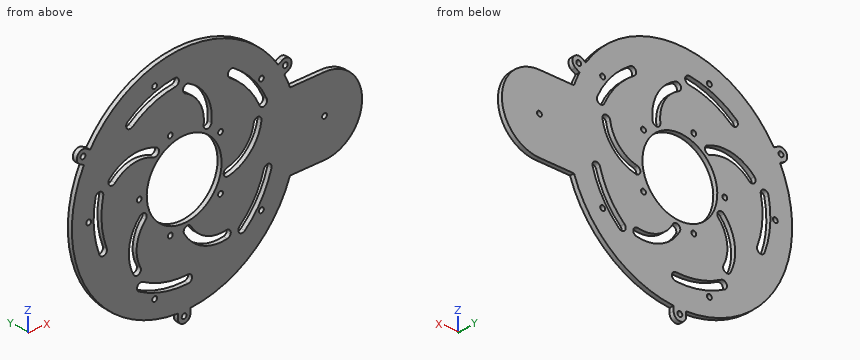
from build123d import *

# Parameters (mm, degrees)
SKETCH1_R           = 50.8
SKETCH1_R_2         = 3.3
BOSS_EXTRUDE1_DEPTH = 6


with BuildPart() as part:
    # Sketch1 → Boss-Extrude1 (new body)
    with BuildSketch(Plane(origin=(0, 0, 0), x_dir=(1, 0, 0), z_dir=(0, 1, 0))):
        with BuildLine():
            Line((190.5, 50.961251532), (143.626985077, 50.961251532))
            ThreePointArc((143.626985077, 50.961251532), (91.342451877, 121.993100154), (8.463835644, 152.16479056))
            Line((8.463835644, 152.16479056), (8.463835644, 158.450241569))
            ThreePointArc((8.463835644, 158.450241569), (0, 166.914077214), (-8.463835644, 158.450241569))
            Line((-8.463835644, 158.450241569), (-8.463835644, 152.16479056))
            ThreePointArc((-8.463835644, 152.16479056), (-131.982271537, 76.2), (-136.010492009, -68.752498599))
            Line((-136.010492009, -68.752498599), (-141.453852257, -71.895224103))
            ThreePointArc((-141.453852257, -71.895224103), (-144.551831116, -83.457038607), (-132.990016613, -86.555017466))
            Line((-132.990016613, -86.555017466), (-127.546656365, -83.412291961))
            ThreePointArc((-127.546656365, -83.412291961), (0, -152.4), (127.546656365, -83.412291961))
            Line((127.546656365, -83.412291961), (132.990016613, -86.555017466))
            ThreePointArc((132.990016613, -86.555017466), (144.551831116, -83.457038607), (141.453852257, -71.895224103))
            Line((141.453852257, -71.895224103), (136.010492009, -68.752498599))
            ThreePointArc((136.010492009, -68.752498599), (140.101433846, -59.977897881), (143.626985077, -50.961251532))
            Line((143.626985077, -50.961251532), (190.5, -50.961251532))
            ThreePointArc((190.5, -50.961251532), (241.461251532, 0), (190.5, 50.961251532))
        make_face()
        with Locations(Location((0, 0, 0), (0, 0, 270))):
            Circle(SKETCH1_R, mode=Mode.SUBTRACT)
        with Locations(Location((-60.96, 0, 0), (0, 0, 270))):
            Circle(SKETCH1_R_2, mode=Mode.SUBTRACT)
        with Locations(Location((-129.54, 0, 0), (0, 0, 270))):
            Circle(SKETCH1_R_2, mode=Mode.SUBTRACT)
        with Locations(Location((-40.030061451, 123.199861121, 0), (0, 0, 270))):
            Circle(SKETCH1_R_2, mode=Mode.SUBTRACT)
        with Locations(Location((-18.837675977, 57.976405233, 0), (0, 0, 270))):
            Circle(SKETCH1_R_2, mode=Mode.SUBTRACT)
        with Locations(Location((104.800061451, 76.141701582, 0), (0, 0, 270))):
            Circle(SKETCH1_R_2, mode=Mode.SUBTRACT)
        with Locations(Location((49.317675977, 35.83138898, 0), (0, 0, 270))):
            Circle(SKETCH1_R_2, mode=Mode.SUBTRACT)
        with Locations(Location((104.800061451, -76.141701582, 0), (0, 0, 270))):
            Circle(SKETCH1_R_2, mode=Mode.SUBTRACT)
        with Locations(Location((49.317675977, -35.83138898, 0), (0, 0, 270))):
            Circle(SKETCH1_R_2, mode=Mode.SUBTRACT)
        with Locations(Location((-40.030061451, -123.199861121, 0), (0, 0, 270))):
            Circle(SKETCH1_R_2, mode=Mode.SUBTRACT)
        with Locations(Location((-18.837675977, -57.976405233, 0), (0, 0, 270))):
            Circle(SKETCH1_R_2, mode=Mode.SUBTRACT)
        with Locations(Location((0, 158.450241569, 0), (0, 0, 270))):
            Circle(SKETCH1_R_2, mode=Mode.SUBTRACT)
        with Locations(Location((137.221934435, -79.225120785, 0), (0, 0, 270))):
            Circle(SKETCH1_R_2, mode=Mode.SUBTRACT)
        with Locations(Location((-137.221934435, -79.225120785, 0), (0, 0, 270))):
            Circle(SKETCH1_R_2, mode=Mode.SUBTRACT)
        with Locations(Location((190.5, 0, 0), (0, 0, 270))):
            Circle(SKETCH1_R_2, mode=Mode.SUBTRACT)
        with BuildLine():
            ThreePointArc((58.830892873, 91.291374091), (24.932369588, 86.543005761), (0.05734711, 63.029389718))
            ThreePointArc((0.05734711, 63.029389718), (2.138397611, 55.817383614), (9.350403715, 57.898434115))
            ThreePointArc((9.350403715, 57.898434115), (29.532704945, 76.976160876), (57.03620605, 80.828740309))
            ThreePointArc((57.03620605, 80.828740309), (63.164866353, 85.162713788), (58.830892873, 91.291374091))
        make_face(mode=Mode.SUBTRACT)
        with BuildLine():
            ThreePointArc((105.003001903, -27.740917993), (90.011815481, 3.031166961), (59.962233041, 19.422612225))
            ThreePointArc((59.962233041, 19.422612225), (53.746287611, 15.214783136), (57.9541167, 8.998837707))
            ThreePointArc((57.9541167, 8.998837707), (82.334787118, -4.30032961), (94.497857139, -29.26720104))
            ThreePointArc((94.497857139, -29.26720104), (100.513571044, -33.756631898), (105.003001903, -27.740917993))
        make_face(mode=Mode.SUBTRACT)
        with BuildLine():
            ThreePointArc((6.064531223, -108.43620429), (30.697991769, -84.669641553), (37.001350951, -51.025555212))
            ThreePointArc((37.001350951, -51.025555212), (31.078634902, -46.414130505), (26.467210194, -52.336846553))
            ThreePointArc((26.467210194, -52.336846553), (21.35299195, -79.633910737), (1.366681525, -98.916865307))
            ThreePointArc((1.366681525, -98.916865307), (-1.044063117, -106.025459647), (6.064531223, -108.43620429))
        make_face(mode=Mode.SUBTRACT)
        with BuildLine():
            ThreePointArc((-101.254915481, -39.276341869), (-71.039413182, -55.359883256), (-37.094140524, -50.958139641))
            ThreePointArc((-37.094140524, -50.958139641), (-34.538634918, -43.900293346), (-41.596481213, -41.34478774))
            ThreePointArc((-41.596481213, -41.34478774), (-69.137912331, -44.916133883), (-93.653201504, -31.866783781))
            ThreePointArc((-93.653201504, -31.866783781), (-101.158837537, -31.770705837), (-101.254915481, -39.276341869))
        make_face(mode=Mode.SUBTRACT)
        with BuildLine():
            ThreePointArc((-68.643510519, 84.162090061), (-74.602763656, 50.455352088), (-59.926790578, 19.53169291))
            ThreePointArc((-59.926790578, 19.53169291), (-52.424685206, 19.282257101), (-52.175249396, 26.784362472))
            ThreePointArc((-52.175249396, 26.784362472), (-64.082571682, 51.874213354), (-59.24754321, 79.222109818))
            ThreePointArc((-59.24754321, 79.222109818), (-61.475536743, 86.390083594), (-68.643510519, 84.162090061))
        make_face(mode=Mode.SUBTRACT)
        with BuildLine():
            ThreePointArc((-114.933952082, 43.33582753), (-122.475383862, 9.358826678), (-120.183999815, -25.369538378))
            ThreePointArc((-120.183999815, -25.369538378), (-113.894475778, -29.466572649), (-109.797441507, -23.177048612))
            ThreePointArc((-109.797441507, -23.177048612), (-111.890799244, 8.55001686), (-105.001114128, 39.590652631))
            ThreePointArc((-105.001114128, 39.590652631), (-108.094945655, 46.429659058), (-114.933952082, 43.33582753))
        make_face(mode=Mode.SUBTRACT)
        with BuildLine():
            ThreePointArc((5.698276738, 122.700191244), (-28.946201909, 119.373048399), (-61.266763184, 106.46215768))
            ThreePointArc((-61.266763184, 106.46215768), (-63.219704511, 99.214411644), (-55.971958475, 97.261470317))
            ThreePointArc((-55.971958475, 97.261470317), (-26.444609232, 109.056574246), (5.205819475, 112.096178291))
            ThreePointArc((5.205819475, 112.096178291), (10.754054583, 117.151956136), (5.698276738, 122.700191244))
        make_face(mode=Mode.SUBTRACT)
        with BuildLine():
            ThreePointArc((118.455680783, 32.497061084), (104.585647237, 64.417774574), (82.319057786, 91.16677034))
            ThreePointArc((82.319057786, 91.16677034), (74.822549631, 90.784451219), (75.204868752, 83.287943063))
            ThreePointArc((75.204868752, 83.287943063), (95.54713192, 58.850652721), (108.218487502, 29.688595562))
            ThreePointArc((108.218487502, 29.688595562), (114.741316904, 25.974231683), (118.455680783, 32.497061084))
        make_face(mode=Mode.SUBTRACT)
        with BuildLine():
            ThreePointArc((67.511360147, -102.615902959), (93.583686637, -79.560674233), (112.142738818, -50.117994966))
            ThreePointArc((112.142738818, -50.117994966), (109.462583308, -43.106535141), (102.451123483, -45.786690651))
            ThreePointArc((102.451123483, -45.786690651), (85.495984285, -72.684870605), (61.676884013, -93.747617155))
            ThreePointArc((61.676884013, -93.747617155), (60.159979178, -101.098998124), (67.511360147, -102.615902959))
        make_face(mode=Mode.SUBTRACT)
        with BuildLine():
            ThreePointArc((-76.731365586, -95.917176899), (-46.747748103, -113.588975417), (-13.011033605, -122.141394676))
            ThreePointArc((-13.011033605, -122.141394676), (-7.17095265, -117.425755073), (-11.886592254, -111.585674118))
            ThreePointArc((-11.886592254, -111.585674118), (-42.70770773, -103.772373223), (-70.100076862, -87.627809328))
            ThreePointArc((-70.100076862, -87.627809328), (-77.56040501, -88.456848752), (-76.731365586, -95.917176899))
        make_face(mode=Mode.SUBTRACT)
    extrude(amount=BOSS_EXTRUDE1_DEPTH)


solid = part.part
Could you check a few things on this model? Use its own coordinates, in mm. Give positions to 0.01 mm unless a question says otherwise; leave off trailing zeros. Loops run counter-clockwise (first coordinate to the right, second up) from the corner with the lowest first, then second, coordinate; pieces in that order, holes last. Notation, with made-up numbers: (51, 58.5) -> (80, 58.5) arc R16 ccw to (80, 80.5) -> close; hole circle Ø3 at (36.5, 40.25). An arc over 180 degrees is marked (long way). Return JSON: item names as keys, results as strings.
Item 1: If we section it at B-B on z = -131.5: List the corners of the cut face in (x, y) for me, plus the area to 3 significant figures.
Geometry results:
{"outline": "(-77.03, 0) -> (77.03, 0) -> (77.03, 6) -> (-77.03, 6) -> close", "area": "924 mm²"}
Item 2: I need wall thicknesses on L1, parallel to X at y = 3.4, z = 15; L2, parallel to Z at x = 101, y = 1.35; L3, parallel to Z at x = -19.5, y = 3.5. Which ranges of each line are inside material? Lowest first, please. Write a range as from..to.
Geometry results:
{"L1": "x = -151.66..-121.91, -111.21..-48.53, 48.53..89.94, 101.59..239.2", "L2": "z = -114.13..-69.91, -48.9..13.58, 33.66..48.9, 69.91..114.13", "L3": "z = -151.15..-121.27, -110.51..-61.21, -54.74..-46.91, 46.91..54.74, 61.21..110.51, 121.27..151.15"}
Item 3: I'm going to push flat-ended pins straight in: pin 1 (4 mm diameter, centred on x = -18.84, z = 57.98, fed in from -Y); pin 2 (1 mm diameter, centred on y = 4, z = 80, fed in from -X); pin 3 (1 mm diameter, centred on x = -14.5, y = 4.5, fed in from +Z); pin 4 (2 mm diameter, centred on y = 5, z = -66, fed in from -X). Where does each tip first touch, or does it pass through?
Geometry results:
{"pin 1": "passes through", "pin 2": "stops at x = -145.68", "pin 3": "stops at z = 151.76", "pin 4": "stops at x = -137.84"}
Item 4: If we section it at A-A on y = 2.85: Count the separate pieces of the cut face and the enclosed holes in it, plus the area to 3 significant figures.
Geometry results:
{"separate pieces": "1", "enclosed holes": "25", "area": "65,500 mm²"}
